from build123d import *

# Parameters (mm, degrees)
F0_W     = 96.003198
F0_H     = 57.444536
F1_DEPTH = 12.7
F2_R     = 10.229848
F3_DEPTH = 25.4


with BuildPart() as f1:
    # F0 (on Front) → F1 (new body, symmetric)
    with BuildSketch(Plane.XZ):
        Rectangle(F0_W, F0_H)
    extrude(amount=F1_DEPTH, both=True)

    # F2 (on face) → F3 (join)
    with BuildSketch(Plane.XZ.offset(12.7)):
        with Locations((-24.000801, -11.410213)):
            Circle(F2_R)
    extrude(amount=F3_DEPTH)


solid = f1.part
Check sheet for the modelled part. Datum: model origin and axes. Units: mm. A direction names the side the tool comes from. Give positions to 0.01 mm unless a question says otherwise; leave off trailing zeros. Loops run counter-clockwise (first coordinate to the right, second up) from the corner with the lowest first, then second, coordinate; pieces in that order, holes last. Notation, with made-up numbers: M -24.5,53 L 10.5,53 A11 cw 10.5,62 Z; hole C 8.5,37.5 d6. An arc over 180 degrees is marked long. Answer as a JSON object with one key per item and string values. Group by question number.
Q1. Cross-section at D-D on y = -28.5. Record the cut outline in (x, z), then the cut area to 3 significant figures.
Q2. Cross-section at C-C on z = -4. Record the cut outline in (x, y).
Q3. Cross-section at B-B on x = -3.5. Record the cut outline in (y, z), then the cut area to 3 significant figures.
Q4. Material ranges on line 1 along Y through (x, z) = (-27.5, 19.5); line 2 along Z through (x, y) = (-25, -19.5); line 3 along X through (y, z) = (-32.5, -19.5), recorded low to high. Write a range as [from, to].
Q5. Cross-section at A-A on z = -25. Record the cut outline in (x, y).
Q6. Go/stop test with flat-tipped pins: P1, Ø5, axis at y = -28, z = -20, coming from the -X side; P2, Ø3, axis at x = -19.5, y = -27.5, coming from the +Z side; P3, Ø10, axis at x = -15, y = -22, coming from the -Z side. Record where each tip stops, or that it passes through.
Q7. Access from +Z, -Z, +X, -X, +Y, -Y to the whole of each face (thin tool, end or side, straight path). Record for faces 1 (the cylindrical face through (-14.55, -25.22, -15.33)), 2 (the flat face through (-24, -38.1, -11)).
Evaluation:
{
 "1": {"outline": "C -24,-11.41 d20.46", "area": "329 mm2"},
 "2": {"outline": "M -48,-12.7 L -31.05,-12.7 L -31.05,-38.1 L -16.95,-38.1 L -16.95,-12.7 L 48,-12.7 L 48,12.7 L -48,12.7 Z"},
 "3": {"outline": "M -12.7,-28.72 L 12.7,-28.72 L 12.7,28.72 L -12.7,28.72 Z", "area": "1,460 mm2"},
 "4": {"line 1": "y = [-12.7, 12.7]", "line 2": "z = [-21.59, -1.23]", "line 3": "x = [-30.26, -17.74]"},
 "5": {"outline": "M -48,-12.7 L 48,-12.7 L 48,12.7 L -48,12.7 Z"},
 "6": {"P1": "stops at x = -32.22", "P2": "stops at z = -1.63", "P3": "stops at z = -20.83"},
 "7": {"face 1": "-Y", "face 2": "+Z, -Z, +X, -X, -Y"}
}
